Read the model definition and answer for the solid it produces. Units are mm, in the model's axes. Face numbers are marked on the shaded views. A direction names the side the tool comes from. Coordinates: 2 decimals unless noted, no trailing zeros. Write each loop counter-clockwise with the first axis right and the second up, starting at its lowest first coordinate (ties: lowest second). Pieces come first, ordered by that corner, then holes.
Item 1: A tool of negligible diameter and unlimited length cuts with its end or side. For the marked faces 4 and 5, from which of +Z, -Z, +X, -X, +Y, -Y can it reach the whole face along a straight path? Write none if from no direction.
Item 2: Section C-C (x = 10) is taken. Give the vertices of the cut face in (y, z).
Item 3: Straight lines are drawn through the part: probe 1 along X at (y, z) = (-3, -7.5); probe 2 along Z at (x, y) = (-13.5, -3); probe 3 along Y at (x, z) = (-9.5, 1). For each, find the intervals that lie inside material, in ascending order.
Item 4: Section A-A (y = -32.5) is taken. Give the vertices of the cut face in (x, z).
Item 5: Section B-B (z = 7) is taken. Give the vertices of the cut face in (x, y), then the cut area to 3 significant figures.
Item 6: Determine the mould class of the marked faces 1, 2 and 3 for opening direction X: released by +X, released by -X, zero draft, split by the parting line, or undercut.
from build123d import *

# Parameters (mm, degrees)
F0_W     = 76.5245743096
F0_H     = 53.4645225853
F0_W_2   = 54.4477272779
F0_H_2   = 5.311973393
F0_H_3   = 5.5775716901
F1_DEPTH = 50.8
F2_W     = 54.4477272779
F2_H     = 2.6621837169
F3_DEPTH = 30.6


with BuildPart() as f1:
    # F0 (on Front) → F1 (new body)
    with BuildSketch(Plane.XZ):
        with Locations((0.4114229232, -2.8822431341)):
            Rectangle(F0_W, F0_H)
        Polygon((-26.0286685079, 12.615935877), (-26.0286685079, 17.9279092699), (28.4190587699, 17.9279092699), (28.4190587699, 12.615935877), (28.4190587699, -15.0063242763), (28.4190587699, -20.5838959664), (-26.0286685079, -20.5838959664), (-26.0286685079, -15.0063242763), align=None, mode=Mode.SUBTRACT)
        with Locations((1.195195131, 15.2719225734)):
            Rectangle(F0_W_2, F0_H_2)
        with Locations((1.195195131, -17.7951101214)):
            Rectangle(F0_W_2, F0_H_3)
    extrude(amount=F1_DEPTH)

    # F2 (on face) → F3 (join)
    with BuildSketch(Plane(origin=(0, 0, 12.615935877), x_dir=(1, 0, 0), z_dir=(0, 0, -1))):
        with Locations((1.195195131, 1.3310918584)):
            Rectangle(F2_W, F2_H)
    extrude(amount=F3_DEPTH)


solid = f1.part
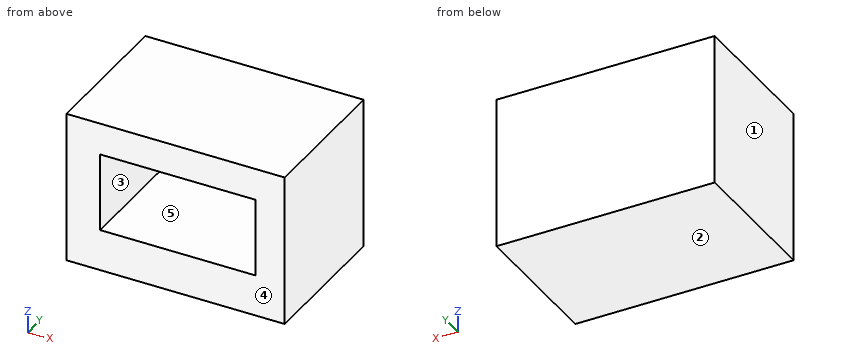
Established:
1. face 4: +Z, -Z, +X, -X, -Y
1. face 5: -Y
2. outline: (-50.8, -29.61) - (0, -29.61) - (0, 23.85) - (-50.8, 23.85) - (-50.8, 12.62) - (-2.66, 12.62) - (-2.66, -15.01) - (-50.8, -15.01) - close
3. probe 1: x = -37.85 to -26.03, 28.42 to 38.67
3. probe 2: z = -29.61 to -15.01, 12.62 to 23.85
3. probe 3: y = -2.66 to 0
4. outline: (-37.85, -29.61) - (38.67, -29.61) - (38.67, 23.85) - (-37.85, 23.85) - close; hole (-26.03, -15.01) - (28.42, -15.01) - (28.42, 12.62) - (-26.03, 12.62) - close
5. outline: (-37.85, -50.8) - (-26.03, -50.8) - (-26.03, -2.66) - (28.42, -2.66) - (28.42, -50.8) - (38.67, -50.8) - (38.67, 0) - (-37.85, 0) - close
5. area: 1,270 mm2
6. face 1: released by -X
6. face 2: zero draft
6. face 3: undercut
